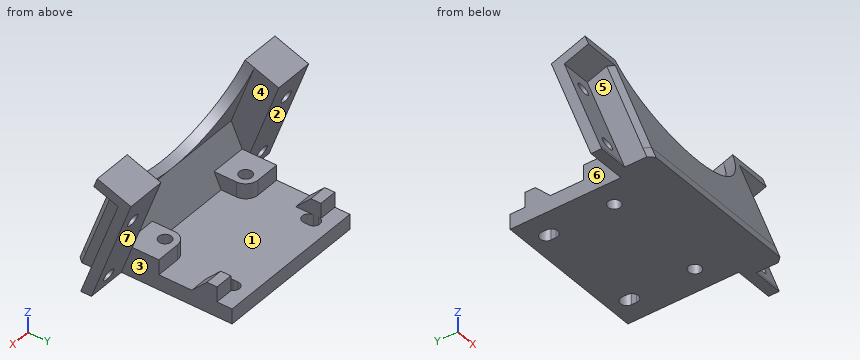
```python
from build123d import *

# Parameters (mm, degrees)
BOSS_EXTRUDE1_DEPTH             = 3
BOSS_EXTRUDE2_REACH             = 67.424
BOSS_EXTRUDE2_DIRECTION_2_REACH = 67.424
BOSS_EXTRUDE3_DEPTH             = 1.8
BOSS_EXTRUDE4_DEPTH             = 6
SKETCH5_R                       = 1.2500000000000013
CUT_EXTRUDE1_DEPTH              = 52.534261642227
BOSS_EXTRUDE5_START             = -17.153882977
BOSS_EXTRUDE5_DEPTH             = 34.307765954
BOSS_EXTRUDE5_START_2           = -23.153882977
BOSS_EXTRUDE5_2_DEPTH           = 46.307765954
SKETCH7_R                       = 1.2499999999999996
CUT_EXTRUDE2_DEPTH              = 72.76321538065721
SKETCH8_R                       = 1.2499999999999996
SKETCH8_W                       = 3.603882977174097
SKETCH8_H                       = 2
BOSS_EXTRUDE6_DEPTH             = 3
CHAMFER1_SIZE                   = 3
CHAMFER3_SIZE                   = 1
CUT_EXTRUDE3_DEPTH              = 54.0045843552169


# Read off the part's stored shape, not the designer's step: Boss-Extrude5
with BuildPart() as part:
    # Sketch1 → Boss-Extrude1 (new body)
    with BuildSketch(Plane.XY):
        Polygon((15.353882977174102, 43.52586008583906), (-15.3538829771741, 43.52586008583904), (-15.3538829771741, 63.52586008583905), (15.3538829771741, 63.52586008583905), align=None)
    extrude(amount=BOSS_EXTRUDE1_DEPTH)

    # Boss-Extrude2: up to this face of the body (flat: up to its plane)
    boss_extrude2_end = Plane(part.part.faces().sort_by_distance((15.353882977, 53.525860086, 1.5))[0])
    # Sketch2 → Boss-Extrude2 (add, up to the picked face)
    with BuildSketch(Plane(origin=(0, 0, 0), x_dir=(0, 0, -1), z_dir=(1, 0, 0)), mode=Mode.PRIVATE) as boss_extrude2_sk1:
        Polygon((-3, 43.52586008583906), (0, 43.52586008583906), (0, 41.52586008583906), (-2.4353936802444784, 34.83467094188486), (-24.048323958320367, 42.701134238375246), (-23.36428367166903, 44.580519479947064), (-10.656874598929635, 39.95540082282564), align=None)
    boss_extrude2_tool1 = split(extrude(boss_extrude2_sk1.sketch, amount=BOSS_EXTRUDE2_REACH, mode=Mode.PRIVATE), bisect_by=boss_extrude2_end, keep=Keep.BOTH, mode=Mode.PRIVATE)
    add(boss_extrude2_tool1.solids().sort_by(Axis((0, 40.026068, 8.762362), (1, 0, 0)))[0])

    # Boss-Extrude2 direction 2: up to this face of the body (flat: up to its plane)
    boss_extrude2_direction_2_end = Plane(part.part.faces().sort_by_distance((-15.353882977, 53.525860086, 1.5))[0])
    # Sketch2 → Boss-Extrude2 direction 2 (add, up to the picked face)
    with BuildSketch(Plane(origin=(0, 0, 0), x_dir=(0, 0, -1), z_dir=(1, 0, 0)), mode=Mode.PRIVATE) as boss_extrude2_direction_2_sk1:
        Polygon((-3, 43.52586008583906), (0, 43.52586008583906), (0, 41.52586008583906), (-2.4353936802444784, 34.83467094188486), (-24.048323958320367, 42.701134238375246), (-23.36428367166903, 44.580519479947064), (-10.656874598929635, 39.95540082282564), align=None)
    boss_extrude2_direction_2_tool1 = split(extrude(boss_extrude2_direction_2_sk1.sketch, amount=-BOSS_EXTRUDE2_DIRECTION_2_REACH, mode=Mode.PRIVATE), bisect_by=boss_extrude2_direction_2_end, keep=Keep.BOTH, mode=Mode.PRIVATE)
    add(boss_extrude2_direction_2_tool1.solids().sort_by(Axis((0, 40.026068, 8.762362), (-1, 0, 0)))[0])

    # Sketch3 → Boss-Extrude3 (add)
    with BuildSketch(Plane(origin=(15.353882977174106, 1.33e-15, 0), x_dir=(0, 0, -1), z_dir=(1, 9e-17, 0))):
        Polygon((-24.048323958320367, 42.701134238375246), (-2.4353936802444798, 34.83467094188486), (3.04e-15, 41.52586008583906), (-21.61293027807589, 49.392323382329444), align=None)
    boss_extrude3 = extrude(amount=BOSS_EXTRUDE3_DEPTH)

    # Sketch4 → Boss-Extrude4 (add)
    with BuildSketch(Plane(origin=(17.1538829771741, 0, 0), x_dir=(0, 0, -1), z_dir=(1, 0, 0))):
        Polygon((-24.048323958320367, 42.701134238375246), (-21.61293027807589, 49.392323382329444), (2.6e-15, 41.52586008583906), (-0.6840402866513355, 39.64647484426724), (-20.41758532315541, 46.82889785410629), (-22.168938716748553, 42.01709395172391), align=None)
    boss_extrude4 = extrude(amount=BOSS_EXTRUDE4_DEPTH)

    # Mirror1: Boss-Extrude3, Boss-Extrude4 across plane
    add(boss_extrude3.mirror(Plane(origin=(0, 0, 0), x_dir=(0, 0, 1), z_dir=(1, 0, 0))))
    add(boss_extrude4.mirror(Plane(origin=(0, 0, 0), x_dir=(0, 0, 1), z_dir=(1, 0, 0))))

    # Sketch5 → Cut-Extrude1 (cut, through all)
    with BuildSketch(Plane(origin=(3.18e-15, 36.66825722516614, -13.34615417237709), x_dir=(1, -8e-17, 3e-17), z_dir=(0, 0.9396926207859083, -0.3420201433256693))):
        with Locations(Location((-20.000000000000004, -31.20268061828034, 0), (0, 0, 270))):
            Circle(SKETCH5_R)
        with Locations(Location((-20.000000000000004, -17.20268061828034, 0), (0, 0, 270))):
            Circle(SKETCH5_R)
        with Locations(Location((19.999999999999996, -17.202680618280336, 0), (0, 0, 270))):
            Circle(SKETCH5_R)
        with Locations(Location((19.999999999999996, -31.202680618280336, 0), (0, 0, 270))):
            Circle(SKETCH5_R)
    extrude(amount=-CUT_EXTRUDE1_DEPTH, mode=Mode.SUBTRACT)

    # Boss-Extrude5 outline → Boss-Extrude5 (add)
    with BuildSketch(Plane.YZ.offset(BOSS_EXTRUDE5_START)):
        Polygon((41.525860086, 0), (34.834670942, 2.43539368), (33.948260134, 0), align=None)
    extrude(amount=BOSS_EXTRUDE5_DEPTH)

    # Boss-Extrude5 2 outline → Boss-Extrude5 2 (add)
    with BuildSketch(Plane.YZ.offset(BOSS_EXTRUDE5_START_2)):
        Polygon((39.397504541, 0), (41.525860086, 0), (39.646474844, 0.684040287), align=None)
    extrude(amount=BOSS_EXTRUDE5_2_DEPTH)

    # Sketch7 → Cut-Extrude2 (cut, through all)
    with BuildSketch(Plane(origin=(0, 0, 0), x_dir=(-1, 0, 0), z_dir=(0, 0, -1))):
        with Locations((-10.500000000000007, 46.525860085839064)):
            Circle(SKETCH7_R)
        with Locations((10.499999999999993, 46.52586008583907)):
            Circle(SKETCH7_R)
        with BuildLine():
            Line((-11.750000000000007, 59.02586008583907), (-11.750000000000007, 60.02586008583906))
            ThreePointArc((-11.750000000000007, 60.02586008583906), (-10.500000000000009, 61.27586008583905), (-9.250000000000016, 60.02586008583906))
            Line((-9.250000000000016, 60.02586008583906), (-9.250000000000016, 59.02586008583907))
            ThreePointArc((-9.250000000000016, 59.02586008583907), (-10.500000000000009, 57.77586008583907), (-11.750000000000007, 59.02586008583907))
        make_face()
        with BuildLine():
            Line((9.249999999999991, 59.02586008583907), (9.249999999999991, 60.02586008583906))
            ThreePointArc((9.249999999999991, 60.02586008583906), (10.499999999999984, 61.27586008583906), (11.749999999999982, 60.02586008583906))
            Line((11.749999999999982, 60.02586008583906), (11.749999999999982, 59.02586008583907))
            ThreePointArc((11.749999999999982, 59.02586008583907), (10.499999999999995, 57.77586008583907), (9.249999999999991, 59.02586008583907))
        make_face()
    extrude(amount=-CUT_EXTRUDE2_DEPTH, mode=Mode.SUBTRACT)

    # Sketch8 → Boss-Extrude6 (add)
    # profile 1 of 2: a face of its own
    with BuildSketch(Plane.XY.offset(3)):
        with BuildLine():
            Line((15.353882977174102, 48.97586008583905), (10.500000000000007, 48.97586008583905))
            ThreePointArc((10.500000000000007, 48.97586008583905), (8.767588386092974, 48.258271699746096), (8.050000000000013, 46.525860085839064))
            Line((8.050000000000013, 46.525860085839064), (8.050000000000015, 40.525860085839064))
            Line((8.050000000000015, 40.525860085839064), (15.353882977174102, 40.525860085839064))
            Line((15.353882977174102, 40.525860085839064), (15.353882977174102, 48.97586008583905))
        make_face()
        with Locations(Location((10.500000000000007, 46.525860085839064, 0), (0, 0, 180))):
            Circle(SKETCH8_R, mode=Mode.SUBTRACT)
    # profile 2 of 2: a face of its own
    with BuildSketch(Plane.XY.offset(3)):
        with Locations((13.551941488587055, 59.52586008583907)):
            Rectangle(SKETCH8_W, SKETCH8_H)
    boss_extrude6 = extrude(amount=BOSS_EXTRUDE6_DEPTH)

    # Mirror2: Boss-Extrude6 across plane
    add(boss_extrude6.mirror(Plane(origin=(0, 0, 0), x_dir=(0, 0, 1), z_dir=(1, 0, 0))))

    # Chamfer1
    chamfer1_edges = [part.edges().sort_by_distance(p)[0] for p in [
        (13.551941488587055, 58.525860085839064, 3),
        (-13.551941488587055, 58.525860085839064, 3),
    ]]
    chamfer(chamfer1_edges, length=CHAMFER1_SIZE - 0.0001)  # a hair under: the kernel refuses the full size

    # Chamfer3
    chamfer3_edges = [part.edges().sort_by_distance(p)[0] for p in [
        (17.153882977174103, 38.42588244680438, 12.302166198496515),
        (-17.1538829771741, 38.42588244680438, 12.302166198496515),
    ]]
    chamfer(chamfer3_edges, length=CHAMFER3_SIZE)

    # Sketch9 → Cut-Extrude3 (cut, through all)
    with BuildSketch(Plane(origin=(0, 31.856453322783743, -11.59480077878396), x_dir=(1, 0, 0), z_dir=(0, 0.9396926207859083, -0.3420201433256693))):
        with BuildLine():
            Line((15.353882977174102, -37.20268061828036), (-15.3538829771741, -37.20268061828037))
            ThreePointArc((-15.3538829771741, -37.20268061828037), (-4.5e-16, -23.67973833731235), (15.353882977174102, -37.20268061828036))
        make_face()
    extrude(amount=-CUT_EXTRUDE3_DEPTH, mode=Mode.SUBTRACT)


solid = part.part
```
The listing builds one solid part. Answer for the finished solid, in the listing's coordinates (mm). Face numbers are marked on the shaded views. A direction names the side the tool comes from. Round coordinates to 2 decimals unless told otherwise and drop trailing zeros. Loops run counter-clockwise (first coordinate to the right, second up) from the corner with the lowest first, then second, coordinate; pieces in that order, holes last. Notation, with made-up numbers: (-31, 76.25) - (-24, 76.25) arc R14 ccw to (-24, 84.25) - close; hole circle Ø6 at (66.25, -11). An arc over 180 degrees is marked (long way). Return JSON: item names as keys, results as strings. Group by question number.
1. Consider probe 1 along Y at (x, z) = (-10.5, 2.1); probe 2 along Y at (x, z) = (-10.5, 2.8); probe 3 along X at (y, z) = (46.25, 13.75). Determine where each line is inside the solid, lowest interval first.
2. The mould has two halves that part along X. Classify the marked faces 1, 2, 3 and 4: pulls with the +X half, pulls with the -X half, needs draft (parallel to the pull), parting line crosses it, or undercut.
3. The part is cut by section A-A on x = 18. Determine the outline of the cut face in (y, z), then the cut area to 3 significant figures.
4. Each of these flat-tipped pins is pushed along its axis until it touches: P1, Ø2, axis at y = 44, z = 19, coming from the +X side; P2, Ø2, axis at x = -6.5, z = 6, coming from the +Y side; P3, Ø1.6, axis at x = -13, y = 59, coming from the +Z side; P4, Ø2, axis at x = 10.5, y = 46.53, coming from the +Z side. Where does it stop, or does it pass through?
5. The part is cut by section B-B on z = 16. State how many separate pieces and enclosed holes the cut face has, then the cut area to 3 significant figures.
6. Which of the six approach directions +Z, -Z, +X, -X, +Y, -Y give full straight-line access (tool end or side, diameter ignored) to the marked faces 5, 6 and 7?
Resolved:
{
 "1": {"probe 1": "y = 34.71 to 45.28, 47.78 to 57.78, 61.28 to 63.53", "probe 2": "y = 34.97 to 45.28, 47.78 to 57.78, 61.28 to 63.53", "probe 3": "x = -23.15 to -15.35, 15.35 to 23.15"},
 "2": {"face 1": "undercut", "face 2": "needs draft", "face 3": "pulls with the +X half", "face 4": "undercut"},
 "3": {"outline": "(39.4, 0) - (41.53, 0) - (49.39, 21.61) - (42.7, 24.05) - (42.02, 22.17) - (46.83, 20.42) - close", "area": "57.0 mm²"},
 "4": {"P1": "stops at x = 17.15", "P2": "stops at y = 42.59", "P3": "stops at z = 6", "P4": "passes through"},
 "5": {"separate pieces": "4", "enclosed holes": "0", "area": "57.3 mm²"},
 "6": {"face 5": "-X, -Y", "face 6": "-Z, -X, +Y", "face 7": "-Z, +X, +Y"}
}
